Autodesk Inventor part; units mm, degrees
ref_plane "YZ Plane" through (0, 0, 0) normal (1, 0, 0) x (0, 1, 0)
ref_plane "XZ Plane" through (0, 0, 0) normal (0, 1, 0) x (-1, 0, 0)
ref_plane "XY Plane" through (0, 0, 0) normal (0, 0, 1) x (1, 0, 0)
sketch "Sketch1" plane through (0, 0, 0) normal (0, 1, 0) x (-1, 0, 0)
  line L0 (0, 0) -> (0, -63.881)
  line L1 (0, -63.881) -> (16.891, -63.881)
  line L2 (16.891, -63.881) -> (16.891, 0)
  line L3 (16.891, 0) -> (0, 0)
  line L4 (16.891, 0) -> (24.638, 0)
  line L5 (24.638, 0) -> (24.638, -11.43)
  line L6 (24.638, -11.43) -> (16.891, -11.43)
  line L7 (16.891, -63.881) -> (24.638, -63.881)
  line L8 (24.638, -63.881) -> (24.638, -52.451)
  line L9 (24.638, -52.451) -> (16.891, -52.451)
  dimension "d0" = 63.881
  dimension "d1" = 16.891
  dimension "d2" = 7.747
  dimension "d3" = 11.43
  dimension "d4" = 7.747
  dimension "d5" = 11.43
extrude "Extrusion1" add sketch "Sketch1" along normal blind 1.651 contours L3 L2 L1 L0
hole "Hole3" at (-5.715, 1.651, -32.131) direction (0, -1, 0) diameter 5.334 end through all
sketch "Sketch2" plane through (0, 1.651, 0) normal (0, 1, 0) x (1, 0, 0)
  line L0 (-16.891, 63.881) -> (-16.891, 31.9405)
  line L1 (-16.891, 63.881) -> (-16.891, 0)
  line L2 (-16.891, 31.9405) -> (-16.891, 37.6555)
  line L3 (-16.891, 37.6555) -> (-24.638, 37.6555)
  line L4 (-24.638, 37.6555) -> (-24.638, 26.2255)
  line L5 (-24.638, 26.2255) -> (-16.891, 26.2255)
  line L6 (-16.891, 31.9405) -> (-16.891, 37.6555)
  point P0 (0, 0)
  dimension "d48" = 31.9405
  dimension "d49" = 5.715
  dimension "d50" = 7.747
  dimension "d51" = 11.43
extrude "Extrusion4" add sketch "Sketch2" along normal blind 6.477
hole "Hole5" at (-20.7645, 4.8895, -26.2255) direction (0, 0, -1) diameter 5.08 end through all
sketch "Sketch3" plane through (0, 1.651, 0) normal (0, 1, 0) x (1, 0, 0)
  line L0 (0, 63.881) -> (-16.891, 63.881)
  line L1 (-16.891, 63.881) -> (-16.891, 0)
  line L2 (-16.891, 0) -> (0, 0)
  line L3 (0, 0) -> (0, 63.881)
  line L4 (0, 63.881) -> (-16.891, 63.881)
extrude "Extrusion5" cut sketch "Sketch3" against normal blind 6.35
sketch "Sketch4" plane through (-16.891, 1.651, -37.6555) normal (1, 0, 0) x (0, 0, -1)
  line L0 (0, 0) -> (-11.43, 0)
  line L1 (-5.715, 0) -> (26.0985, 0)
  line L2 (26.0985, 0) -> (26.0985, 1.651)
  line L3 (26.0985, 0) -> (26.0985, 1.651)
  line L4 (26.0985, 1.651) -> (-37.7825, 1.651)
  line L5 (-37.7825, 1.651) -> (-37.7825, 0)
  line L6 (-37.7825, 0) -> (-11.43, 0)
  point P0 (-37.6555, -1.651)
  dimension "d65" = 31.8135
  dimension "d66" = 1.651
  dimension "d67" = 1.651
  dimension "d68" = 63.881
extrude "Extrusion6" add sketch "Sketch4" along normal blind 16.637
hole "Hole6" at (-8.001, 3.302, -8.763) direction (0, -1, 0) diameter 5.334 end through all
hole "Hole7" at (-8.001, 3.302, -54.864) direction (0, -1, 0) diameter 5.334 end through all
hole "Hole8" at (-5.969, 3.302, -31.8135) direction (0, -1, 0) diameter 5.334 end through all
properties part number "door hinge for conveyor part 2"
Can you work these out from the model? Positions are in its coordinate system, mm. A direction names the side the tool comes from. Round coordinates to 2 decimals unless told otherwise and drop trailing zeros. Order: outer loops, then holes, each group sorted by start corner. A loop starts at its lowest first (then second) coordinate and runs counter-clockwise, first axis right, second up.
(1) On a 3-axis mill with a long thin cutter (end or side, diameter ignored), from which of +Z, -Z, +X, -X, +Y, -Y can I reach the whole of each face in a straight line? I mean faces 4 (the face through (-0.254, 2, -31)), 5 (the face through (-16.891, 2, -51)), 6 (the face through (-23.4, 4.1, -26.226)). Say none if no direction works.
Results are:
face 4: +Z, -Z, +X, +Y, -Y
face 5: -Z, -X, +Y, -Y
face 6: +Z, -X, +Y, -Y
(2) We'd pull the mould along X, two halves only. Please class faces 1 (the face through (-10, 1.651, -32)), 2 (the face through (-16.891, 6, -32)), 3 (the face through (-18.51, 3.72, -32.02)): +X half, -X half, draft (parallel to the pull), parting line (faces both ways), or undercut.
Results are:
face 1: draft
face 2: +X half
face 3: undercut
(3) If we section it at B-B (z = -56.5): Please give me the cut outline in (x, y).
Results are:
outline: (-16.89, 1.65) - (-10.11, 1.65) - (-10.11, 3.3) - (-16.89, 3.3) - close; (-5.89, 1.65) - (-0.25, 1.65) - (-0.25, 3.3) - (-5.89, 3.3) - close
(4) If I drill on L1, parallel to Y at x = -8.5, z = -30; L2, parallel to Z at x = -19.75, y = 7.5; L3, parallel to X at y = 6.25, z = -35, over which ranges is the centre line in solid material (lowest first)?
Results are:
L1: y = 1.65 to 3.3
L2: z = -37.66 to -26.23
L3: x = -24.64 to -22.91, -18.62 to -16.89
(5) If we section it at D-D (x = -13.75): Please give me the cut outline in (y, z), plus the area to 3 significant figures.
Results are:
outline: (1.65, -63.75) - (3.3, -63.75) - (3.3, 0.13) - (1.65, 0.13) - close
area: 105 mm2
(6) If we section it at A-A (x = -4.5): Please give me the cut outline in (y, z), plus the area to 3 significant figures.
Results are:
outline: (1.65, -63.75) - (3.3, -63.75) - (3.3, -34.04) - (1.65, -34.04) - close; (1.65, -29.59) - (3.3, -29.59) - (3.3, 0.13) - (1.65, 0.13) - close
area: 98.1 mm2
(7) I'm going to push flat-ended pins straight in: pin 1 (5 mm diameter, centred on x = -7, z = -33, fed in from +Y); pin 2 (1.4 mm diameter, centred on y = 6.5, z = -34.5, fed in from +X); pin 3 (0.8 mm diameter, centred on y = 2.5, z = -16.5, fed in from -X). Where does each tip first touch, or does it pass through?
Results are:
pin 1: stops at y = 3.3
pin 2: stops at x = -16.89
pin 3: stops at x = -16.89
(8) If we section it at C-C (z = -33.5): Please give me the cut outline in (x, y), plus the area to 3 significant figures.
Results are:
outline: (-24.64, 1.65) - (-8.04, 1.65) - (-8.04, 3.3) - (-16.89, 3.3) - (-16.89, 8.13) - (-24.64, 8.13) - close; (-3.9, 1.65) - (-0.25, 1.65) - (-0.25, 3.3) - (-3.9, 3.3) - close; hole circle Ø5.08 at (-20.76, 4.89)
area: 50.6 mm2
